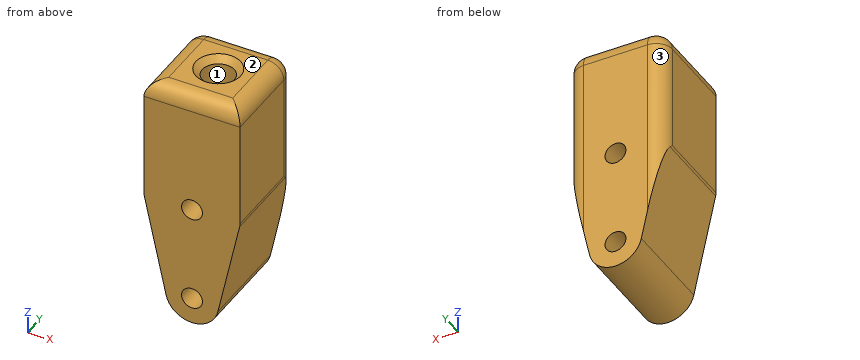
```python
from build123d import *

# Parameters (mm, degrees)
SKETCH2_R           = 2.0701
BOSS_EXTRUDE1_DEPTH = 19.05
SKETCH3_R           = 3.175
CUT_EXTRUDE1_DEPTH  = 19.05
CHAMFER1_SIZE       = 1.27
FILLET1_R           = 3.175


with BuildPart() as part:
    # Sketch2 → Boss-Extrude1 (new body)
    with BuildSketch(Plane(origin=(0, 0, 0), x_dir=(1, 0, 0), z_dir=(0, 1, 0))):
        with BuildLine():
            Line((9.525, -24.2951), (-9.525, -24.2951))
            Line((-9.525, -24.2951), (-9.525, 0))
            Line((-9.525, 0), (-5.12453766, 20.168117963))
            ThreePointArc((-5.12453766, 20.168117963), (0, 24.2951), (5.12453766, 20.168117963))
            Line((5.12453766, 20.168117963), (9.525, 0))
            Line((9.525, 0), (9.525, -24.2951))
        make_face()
        with Locations(Location((0, 0, 0), (0, 0, 90))):
            Circle(SKETCH2_R, mode=Mode.SUBTRACT)
        with Locations(Location((0, 19.05, 0), (0, 0, 90))):
            Circle(SKETCH2_R, mode=Mode.SUBTRACT)
    extrude(amount=BOSS_EXTRUDE1_DEPTH)

    # Sketch3 → Cut-Extrude1 (cut)
    with BuildSketch(Plane.XY.offset(24.2951)):
        with Locations((0, 9.525)):
            Circle(SKETCH3_R)
    extrude(amount=-CUT_EXTRUDE1_DEPTH, mode=Mode.SUBTRACT)

    # Chamfer1
    chamfer1_edges = [part.edges().sort_by_distance(p)[0] for p in [
        (-3.175, 9.525, 24.2951),
    ]]
    chamfer(chamfer1_edges, length=CHAMFER1_SIZE)

    # Fillet1
    fillet1_edges = [part.edges().sort_by_distance(p)[0] for p in [
        (9.525, 9.525, 0),
        (9.525, 9.525, 24.2951),
        (-9.525, 9.525, 24.2951),
        (-9.525, 9.525, 0),
        (-9.525, 19.05, 12.14755),
        (0, 19.05, 24.2951),
        (9.525, 19.05, 12.14755),
        (0, 0, 24.2951),
    ]]
    fillet(fillet1_edges, radius=FILLET1_R)


solid = part.part
```
Check sheet for the modelled part. Datum: model origin and axes. Units: mm. Face numbers are marked on the shaded views. Coordinates: 2 decimals unless noted, no trailing zeros. Loops run counter-clockwise (first coordinate to the right, second up) from the corner with the lowest first, then second, coordinate; pieces in that order, holes last.
1) Sectioned sample at B-B (x = 0). Record the boundary of the cut face in (y, z) (3 decimals), and give its area (3 significant figures).
2) Sectioned sample at A-A (z = 10.5). Record the boundary of the cut face in (x, y) (3 decimals).
3) Sectioned sample at C-C (z = -19.05). Record the boundary of the cut face in (x, y), and give its area (3 significant figures).
4) Material ranges on probe 1 along Z at (x, y) = (-0.5, 8); probe 2 along Z at (x, y) = (-1.5, 4.25); probe 3 along X at (y, z) = (7.25, -19.05), recorded low to high.
5) Gauge pin test, flat ends, axial feed: pin 1 (4 mm diameter, centred on y = 11.5, z = -4.5, fed in from +X); pin 2 (3 mm diameter, centred on x = -1.5, y = 10.5, fed in from +Z); pin 3 (2.5 mm diameter, centred on x = 0, z = 0, fed in from +Y); pin 4 (8 mm diameter, centred on y = 8, z = -19.5, fed in from -X). Record the tip position at first contact, or that the pin passes through.
6) Sectioned sample at D-D (y = 12). Count the separate pieces of the cut face and the enclosed holes in it, and give its area (3 significant figures).
7) Release check for a two-part mould opening along Y. For the marked faces 1, 2 and 3 record: released by +Y, released by -Y, zero draft, split by the parting line, or undercut.
Check sheet entries:
1. outline: (0, -24.295) - (19.05, -24.295) - (19.05, -21.12) - (0, -21.12) - close; (0, -16.98) - (19.05, -16.98) - (19.05, -2.07) - (0, -2.07) - close; (0, 2.07) - (19.05, 2.07) - (19.05, 21.12) arc R3.175 ccw to (15.875, 24.295) - (13.97, 24.295) - (12.7, 23.025) - (12.7, 5.245) - (6.35, 5.245) - (6.35, 23.025) - (5.08, 24.295) - (3.175, 24.295) arc R3.175 ccw to (0, 21.12) - close
1. area: 641 mm2
2. outline: (-9.525, 0) - (9.525, 0) - (9.525, 15.875) arc R3.175 ccw to (6.35, 19.05) - (-6.35, 19.05) arc R3.175 ccw to (-9.525, 15.875) - close; hole circle Ø6.35 at (0, 9.525)
3. outline: (-5.37, 0) - (-2.07, 0) - (-2.07, 19.05) - (-5.37, 19.05) - close; (2.07, 0) - (5.37, 0) - (5.37, 19.05) - (2.07, 19.05) - close
3. area: 126 mm2
4. probe 1: z = -24.27 to -21.06, -17.04 to -2.01, 2.01 to 5.25
4. probe 2: z = -24.08 to -20.48, -17.62 to -1.43, 1.43 to 24.3
4. probe 3: x = -5.37 to -2.07, 2.07 to 5.37
5. pin 1: stops at x = 8.98
5. pin 2: stops at z = 23.14
5. pin 3: passes through
5. pin 4: stops at x = -6.14
6. separate pieces: 1
6. enclosed holes: 2
6. area: 681 mm2
7. face 1: undercut
7. face 2: zero draft
7. face 3: released by +Y
